Answer from the drawing. Dimensions are ordinates in mm from the lowest x, y and z of the part. A direction names the side the tool comes from. Coordinates: 2 decimals unless noted, no trailing zeros. Loops run counter-clockwise (first coordinate to the right, second up) from the corner with the lowest first, then second, coordinate; pieces in that order, holes last. Notation, with made-up numbers: (55.25, -29) - (65.25, -29) arc R7 cw to (65.25, -24) - close; hole circle Ø3 at (5.5, 53). An arc over 180 degrees is marked (long way). Write each question's results on one line, items separated by ' | '. Start each with the question number.
1. A cutting plane is placed at C-C on x = 20. Determine the outline of the cut face in (y, z).
2. Find the intervals of material crossed by line 1 along X through (y, z) = (71.9, 20); line 2 along X through (y, z) = (32.5, 17), in increasing order. Write a range as [from, to].
3. Each of these flat-tipped pins is pushed along its axis until it touches: P1, Ø4, axis at y = 33, z = 19, coming from the -X side; P2, Ø6.5, axis at x = 36.25, z = 20, coming from the -Y side; P3, Ø7.5, axis at x = 10, y = 68.5, coming from the -Z side; P4, Ø2, axis at y = 72, z = 19.5, coming from the -X side. Where does it stop, or does it pass through?
4. A cutting plane is placed at A-A on z = 3.75. Determine the outline of the cut face in (x, y), then the cut area to 3 significant figures.
5. Which of the six approach directions +Z, -Z, +X, -X, +Y, -Y give full straight-line access (tool end or side, diameter ignored) to the marked faces 1, 2, 3 and 4?
6. A cutting plane is placed at D-D on x = 3.75. Determine the outline of the cut face in (y, z).
7. A cutting plane is placed at B-B on y = 65.5. Determine the outline of the cut face in (x, z), then the cut area to 3 significant figures.
8. Determine the mould class of the marked faces 5, 6 and 7 for opening direction Z: released by +Z, released by -Z, zero draft, split by the parting line, or undercut.
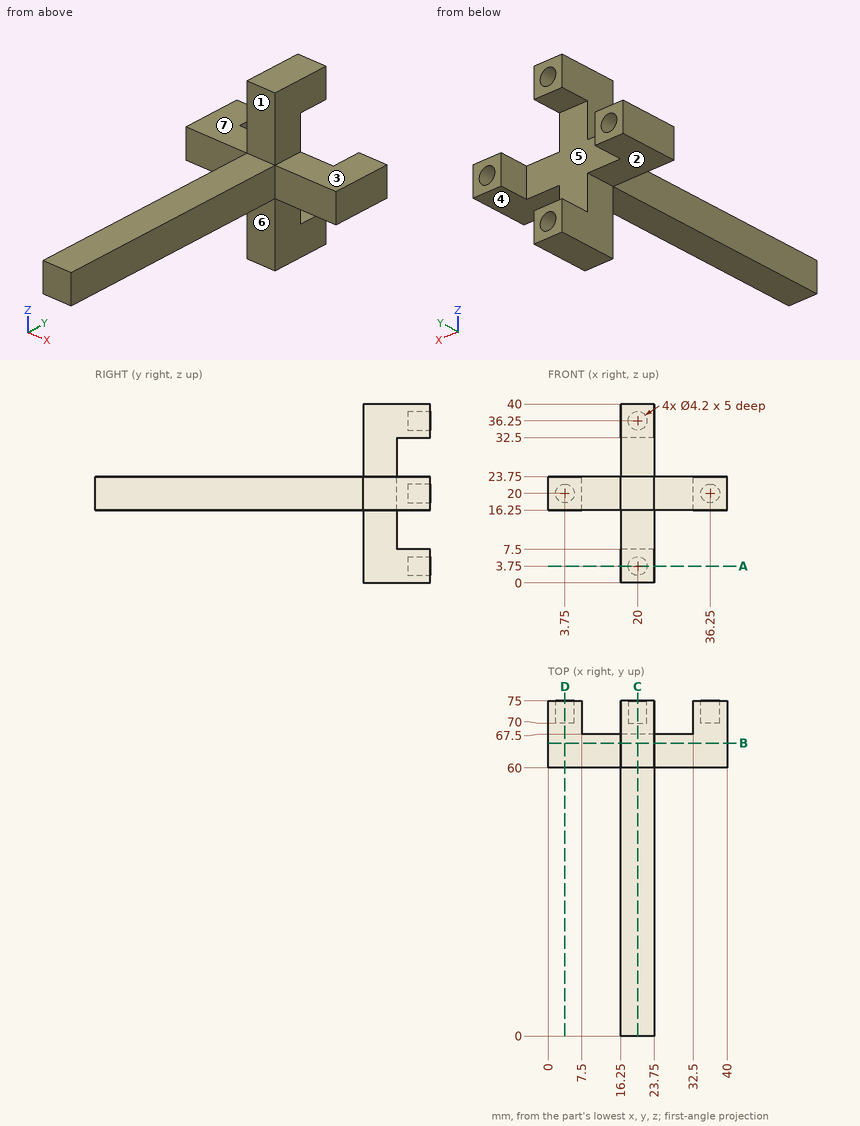
Values:
1) outline: (0, 16.25) - (60, 16.25) - (60, 0) - (75, 0) - (75, 1.65) - (70, 1.65) - (70, 5.85) - (75, 5.85) - (75, 7.5) - (67.5, 7.5) - (67.5, 32.5) - (75, 32.5) - (75, 34.15) - (70, 34.15) - (70, 38.35) - (75, 38.35) - (75, 40) - (60, 40) - (60, 23.75) - (0, 23.75) - close
2) line 1: [0, 1.65], [5.85, 7.5], [32.5, 34.15], [38.35, 40] | line 2: [16.25, 23.75]
3) P1: x = 16.25 | P2: y = 60 | P3: z = 16.25 | P4: x = 0
4) outline: (16.25, 60) - (23.75, 60) - (23.75, 75) - (22.1, 75) - (22.1, 70) - (17.9, 70) - (17.9, 75) - (16.25, 75) - close | area: 91.5 mm^2
5) face 1: +Z, +X, -X, -Y | face 2: -Z, -X, +Y, -Y | face 3: +Z, +X, +Y, -Y | face 4: -Z, +X, +Y, -Y
6) outline: (60, 16.25) - (75, 16.25) - (75, 17.9) - (70, 17.9) - (70, 22.1) - (75, 22.1) - (75, 23.75) - (60, 23.75) - close
7) outline: (0, 16.25) - (16.25, 16.25) - (16.25, 0) - (23.75, 0) - (23.75, 16.25) - (40, 16.25) - (40, 23.75) - (23.75, 23.75) - (23.75, 40) - (16.25, 40) - (16.25, 23.75) - (0, 23.75) - close | area: 544 mm^2
8) face 5: undercut | face 6: zero draft | face 7: released by +Z
